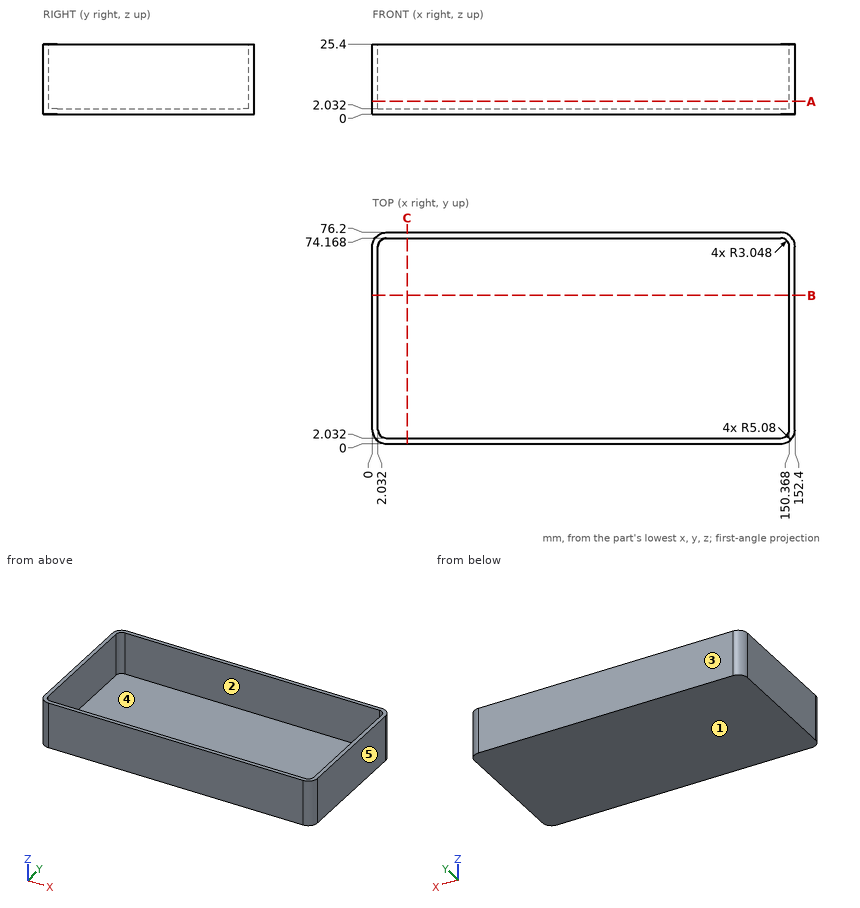
Geometry check sheet. Reference: drawing and pictorial views, mm from the part's lowest x, y, z. A direction names the side the tool comes from. Give positions to 0.01 mm unless a question says otherwise; leave off trailing zeros. Loops run counter-clockwise (first coordinate to the right, second up) from the corner with the lowest first, then second, coordinate; pieces in that order, holes last. Notation, with made-up numbers: (-34.75, 62) - (14.25, 62) arc R21 cw to (14.25, 88) - close; hole circle Ø4 at (-17, 62.5). An arc over 180 degrees is marked (long way). Use CSV: the item, a comma, the result in double quotes. Start each with the question number.
Q1. Release check for a two-part mould opening along X. For the marked faces 3, 4 and 5 record: +X half, -X half, draft (parallel to the pull), parting line (faces both ways), or undercut.
Q2. Section check C-C, the plane x = 12.5. Record the cut outline in (y, z), and give its area (3 significant figures).
Q3. Go/stop test with flat-tipped pins: pin 1 Ø1.5 at (x, y) = (24.5, 22) entering from +Z; pin 2 Ø7 at (y, z) = (38.5, 13) entering from -X. Record where each tip stops, or that it passes through.
Q4. Scan lines: probe 1 along Y at (x, z) = (121.5, 5); probe 2 along X at (y, z) = (48.5, 21); probe 3 along Z at (x, y) = (83, 33). Record each from-to range of solid material in increasing order. Write a range as from..to.
Q5. Section check A-A, the plane z = 4.75. Record the cut outline in (x, y), and give its area (3 significant figures).
Q6. Section check B-B, the plane y = 53.5. Record the cut outline in (x, z), and give its area (3 significant figures).
Q7. Access from +Z, -Z, +X, -X, +Y, -Y to the whole of each face (thin tool, end or side, straight path). Record for the marked faces 1 and 2.
Findings below:
1,face 3,"draft"
1,face 4,"undercut"
1,face 5,"+X half"
2,outline,"(0, 0) - (76.2, 0) - (76.2, 25.4) - (74.17, 25.4) - (74.17, 2.03) - (2.03, 2.03) - (2.03, 25.4) - (0, 25.4) - close"
2,area,"250 mm^2"
3,pin 1,"stops at z = 2.03"
3,pin 2,"stops at x = 0"
4,probe 1,"y = 0..2.03, 74.17..76.2"
4,probe 2,"x = 0..2.03, 150.37..152.4"
4,probe 3,"z = 0..2.03"
5,outline,"(0, 5.08) arc R5.08 ccw to (5.08, 0) - (147.32, 0) arc R5.08 ccw to (152.4, 5.08) - (152.4, 71.12) arc R5.08 ccw to (147.32, 76.2) - (5.08, 76.2) arc R5.08 ccw to (0, 71.12) - close; hole (2.03, 5.08) arc R3.05 ccw to (5.08, 2.03) - (147.32, 2.03) arc R3.05 ccw to (150.37, 5.08) - (150.37, 71.12) arc R3.05 ccw to (147.32, 74.17) - (5.08, 74.17) arc R3.05 ccw to (2.03, 71.12) - close"
5,area,"898 mm^2"
6,outline,"(0, 0) - (152.4, 0) - (152.4, 25.4) - (150.37, 25.4) - (150.37, 2.03) - (2.03, 2.03) - (2.03, 25.4) - (0, 25.4) - close"
6,area,"405 mm^2"
7,face 1,"-Z, +X, -X, +Y, -Y"
7,face 2,"+Z"
